from build123d import *

# Parameters (mm, degrees)
SKETCH2_R               = 60
BOSS_EXTRUDE1_DEPTH     = 35
BOSS_EXTRUDE2_DEPTH     = 15
SKETCH5_R               = 20
BOSS_EXTRUDE3_DEPTH     = 2.5
SKETCH6_R               = 15
BOSS_EXTRUDE4_DEPTH     = 9
BOSS_EXTRUDE5_START     = 2.5
SKETCH7_R               = 20
BOSS_EXTRUDE5_DEPTH     = 2.5
SKETCH8_R               = 15
BOSS_EXTRUDE6_DEPTH     = 9
BOSS_EXTRUDE7_START     = 2.5
SKETCH9_R               = 20
BOSS_EXTRUDE7_DEPTH     = 2.5
CUT_EXTRUDE1_REACH      = 137
SKETCH11_W              = 60
SKETCH11_H              = 10
CUT_EXTRUDE2_DEPTH      = 35
CUT_EXTRUDE3_DEPTH      = 34.5
CUT_EXTRUDE3_DEPTH_BACK = 24.5
SKETCH12_R              = 6
CUT_EXTRUDE4_START      = -17.5
SKETCH15_R              = 60
CUT_EXTRUDE4_DEPTH      = 17.5
SKETCH17_R              = 16
CUT_EXTRUDE6_DEPTH      = 5


with BuildPart() as part:
    # Sketch2 → Boss-Extrude1 (new body)
    with BuildSketch(Plane(origin=(0, 0, 0), x_dir=(1, 0, 0), z_dir=(0, 1, 0))):
        with Locations(Location((0, 0, 0), (0, 0, 270))):
            Circle(SKETCH2_R)
    extrude(amount=BOSS_EXTRUDE1_DEPTH)

    # Sketch4 → Boss-Extrude2 (add, symmetric)
    with BuildSketch(Plane.XY):
        with BuildLine():
            Line((-35, 0), (-35, -35))
            ThreePointArc((-35, -35), (0, -70), (35, -35))
            Line((35, -35), (35, 0))
            Line((35, 0), (-35, 0))
        make_face()
    extrude(amount=BOSS_EXTRUDE2_DEPTH, both=True)

    # Sketch5 → Boss-Extrude3 (add, symmetric)
    with BuildSketch(Plane.XY.offset(15)):
        with Locations((0, -35)):
            Circle(SKETCH5_R)
    boss_extrude3 = extrude(amount=BOSS_EXTRUDE3_DEPTH, both=True)

    # Sketch6 → Boss-Extrude4 (add)
    with BuildSketch(Plane.XY.offset(17.5)):
        with Locations((0, -35)):
            Circle(SKETCH6_R)
    boss_extrude4 = extrude(amount=BOSS_EXTRUDE4_DEPTH)

    # Sketch7 → Boss-Extrude5 (add)
    with BuildSketch(Plane.XY.offset(26.5).offset(BOSS_EXTRUDE5_START)):
        with Locations((0, -35)):
            Circle(SKETCH7_R)
    boss_extrude5 = extrude(amount=-BOSS_EXTRUDE5_DEPTH)

    # Sketch8 → Boss-Extrude6 (add)
    with BuildSketch(Plane.XY.offset(29)):
        with Locations((0, -35)):
            Circle(SKETCH8_R)
    boss_extrude6 = extrude(amount=BOSS_EXTRUDE6_DEPTH)

    # Sketch9 → Boss-Extrude7 (add)
    with BuildSketch(Plane.XY.offset(38).offset(BOSS_EXTRUDE7_START)):
        with Locations((0, -35)):
            Circle(SKETCH9_R)
    boss_extrude7 = extrude(amount=-BOSS_EXTRUDE7_DEPTH)

    # Mirror1: Boss-Extrude3, Boss-Extrude4, Boss-Extrude5, Boss-Extrude6, Boss-Extrude7 across plane
    add(boss_extrude3.mirror(Plane.XY))
    add(boss_extrude4.mirror(Plane.XY))
    add(boss_extrude5.mirror(Plane.XY))
    add(boss_extrude6.mirror(Plane.XY))
    add(boss_extrude7.mirror(Plane.XY))

    # Sketch10 → Cut-Extrude1 (cut, up to next)
    with BuildSketch(Plane(origin=(0, 35, 0), x_dir=(1, 0, 0), z_dir=(0, 1, 0)), mode=Mode.PRIVATE) as cut_extrude1_sk1:
        with BuildLine():
            Line((-35, -17.5), (35, -17.5))
            ThreePointArc((35, -17.5), (40, -22.5), (35, -27.5))
            Line((35, -27.5), (-35, -27.5))
            ThreePointArc((-35, -27.5), (-40, -22.5), (-35, -17.5))
        make_face()
    cut_extrude1_tool1 = extrude(cut_extrude1_sk1.sketch, amount=-CUT_EXTRUDE1_REACH, mode=Mode.PRIVATE) & part.part
    cut_extrude1 = cut_extrude1_tool1.solids().sort_by_distance((0, 35, 22.5))[0]
    add(cut_extrude1, mode=Mode.SUBTRACT)

    # Mirror2: Cut-Extrude1 across plane
    add(cut_extrude1.mirror(Plane.XY), mode=Mode.SUBTRACT)

    # Sketch11 → Cut-Extrude2 (cut)
    with BuildSketch(Plane(origin=(0, 35, 0), x_dir=(1, 0, 0), z_dir=(0, 1, 0))):
        Rectangle(SKETCH11_W, SKETCH11_H)
    extrude(amount=-CUT_EXTRUDE2_DEPTH, mode=Mode.SUBTRACT)

    # Sketch12 → Cut-Extrude3 (cut, two sides: drawn at the far end of the back side and taken through both)
    with BuildSketch(Plane.XY.offset(-5).offset(-CUT_EXTRUDE3_DEPTH_BACK)):
        with Locations(Location((-17.5, 17.5, 0), (0, 0, 180))):
            Circle(SKETCH12_R)
        with Locations(Location((17.5, 17.5, 0), (0, 0, 180))):
            Circle(SKETCH12_R)
    extrude(amount=CUT_EXTRUDE3_DEPTH + CUT_EXTRUDE3_DEPTH_BACK, mode=Mode.SUBTRACT)

    # Sketch15 → Cut-Extrude4 (cut)
    with BuildSketch(Plane(origin=(0, 35, 0), x_dir=(1, 0, 0), z_dir=(0, 1, 0)).offset(CUT_EXTRUDE4_START)):
        with Locations(Location((0, 0, 0), (0, 0, 270))):
            Circle(SKETCH15_R)
    extrude(amount=CUT_EXTRUDE4_DEPTH, mode=Mode.SUBTRACT)

    # Sketch17 → Cut-Extrude6 (cut, symmetric)
    with BuildSketch(Plane.XY.offset(-11.25)):
        with Locations((-17.5, 17.5)):
            Circle(SKETCH17_R)
        with Locations((17.5, 17.5)):
            Circle(SKETCH17_R)
    cut_extrude6 = extrude(amount=CUT_EXTRUDE6_DEPTH, both=True, mode=Mode.SUBTRACT)

    # Mirror3: Cut-Extrude6 across plane
    add(cut_extrude6.mirror(Plane.XY), mode=Mode.SUBTRACT)


solid = part.part
Design review of the part built by this model. Coordinates are the model's own, in mm. A direction names the side the tool comes from. Round coordinates to 2 decimals unless told otherwise and drop trailing zeros. Write each loop counter-clockwise with the first axis right and the second up, starting at its lowest first coordinate (ties: lowest second). Pieces come first, ordered by that corner, then holes. Notation, with made-up numbers: (4.5, -7) -> (18.5, -7) arc R26 cw to (18.5, 12) -> close; hole circle Ø2 at (76.5, 65.25). An arc over 180 degrees is marked (long way). One line per question, with ' | ' between items.
(1) Take a section at A-A, the plane y = -52.5. State the section outline as (x, z) points.
Result sheet:
outline: (-30.31, -15) -> (-9.68, -15) -> (-9.68, -17.5) -> (9.68, -17.5) -> (9.68, -15) -> (30.31, -15) -> (30.31, 15) -> (9.68, 15) -> (9.68, 17.5) -> (-9.68, 17.5) -> (-9.68, 15) -> (-30.31, 15) -> close; (-9.68, -40.5) -> (9.68, -40.5) -> (9.68, -38) -> (-9.68, -38) -> close; (-9.68, -29) -> (9.68, -29) -> (9.68, -26.5) -> (-9.68, -26.5) -> close; (-9.68, 26.5) -> (9.68, 26.5) -> (9.68, 29) -> (-9.68, 29) -> close; (-9.68, 38) -> (9.68, 38) -> (9.68, 40.5) -> (-9.68, 40.5) -> close
(2) Insertion check: P1, Ø2, axis at y = -39.5, z = 5, coming from the -X side; P2, Ø9, axis at x = -12.5, y = 11.5, coming from the +Z side; P3, Ø10, axis at x = 0.5, z = 5.5, coming from the -Y side; P4, Ø6, axis at x = -39, y = -43.5, coming from the +Z side. Each pin has a flat end and moves straight along its axis. Give the tip position at first contact, or say it passes through.
Result sheet:
P1: x = -34.82 | P2: z = 59.46 | P3: y = -70 | P4: through
(3) Take a section at C-C, the plane x = -26. State the section outline as (y, z) points.
Result sheet:
outline: (-58.43, -15) -> (0, -15) -> (0, -17.5) -> (17.5, -17.5) -> (17.5, -16.25) -> (3.94, -16.25) -> (3.94, -6.25) -> (17.5, -6.25) -> (17.5, -5) -> (0, -5) -> (0, 5) -> (17.5, 5) -> (17.5, 6.25) -> (3.94, 6.25) -> (3.94, 16.25) -> (17.5, 16.25) -> (17.5, 17.5) -> (0, 17.5) -> (0, 15) -> (-58.43, 15) -> close; (0, -54.07) -> (17.5, -54.07) -> (17.5, -27.5) -> (0, -27.5) -> close; (0, 27.5) -> (17.5, 27.5) -> (17.5, 54.07) -> (0, 54.07) -> close
(4) Wall thickness on line 1 (Z direction, x = 26, y = 7); line 2 (Z direction, x = -2.5, y = -13.5); line 3 (Y direction, x = 47.5, z = 27.5): over which ranges is each line inside the solid? List them lowest first. Write a range as [from, to].
Result sheet:
line 1: [-54.07, -27.5], [-17.5, -16.25], [-6.25, -5], [5, 6.25], [16.25, 17.5], [27.5, 54.07] | line 2: [-15, 15] | line 3: [0, 17.5]
(5) Take a section at D-D, the plane x = 17.5. State how many separate pieces and enclosed holes the cut face has, and give its area (3 significant figures).
Result sheet:
separate pieces: 7 | enclosed holes: 0 | area: 3,360 mm2
(6) Machinability: for faces 4 (the flat face through (35, -18, 0)), 5 (the cylindrical face through (-2.6, -15.17, 16.27)), 6 (the flat face through (-30, 9, 0)), 7 (the flat face through (3, -20, -38)), which of the approach directions +Z, -Z, +X, -X, +Y, -Y give a long, thin tool a straight path to every point of the face, cutting with its end or side? Answer none if there is none.
Result sheet:
face 4: +Z, -Z, +X, -Y | face 5: +Z | face 6: +Y | face 7: none
(7) Take a section at B-B, the plane z = -23. State the section outline as (x, y) points.
Result sheet:
outline: (-55.42, 0) -> (-39.97, 0) -> (-39.97, 17.5) -> (-55.42, 17.5) -> close; circle Ø30 at (0, -35); (39.97, 0) -> (55.42, 0) -> (55.42, 17.5) -> (39.97, 17.5) -> close
(8) Draft analysis for pull direction Z (two halves, no side actions). For faces 1 (the flat face through (1, 0, -28)), 2 (the flat face through (17, 10, 6.25)), 3 (the cylindrical face through (-1.953, -20.128, -21.937)), state which applies: released by +Z, released by -Z, zero draft, split by the parting line, or undercut.
Result sheet:
face 1: zero draft | face 2: undercut | face 3: undercut
